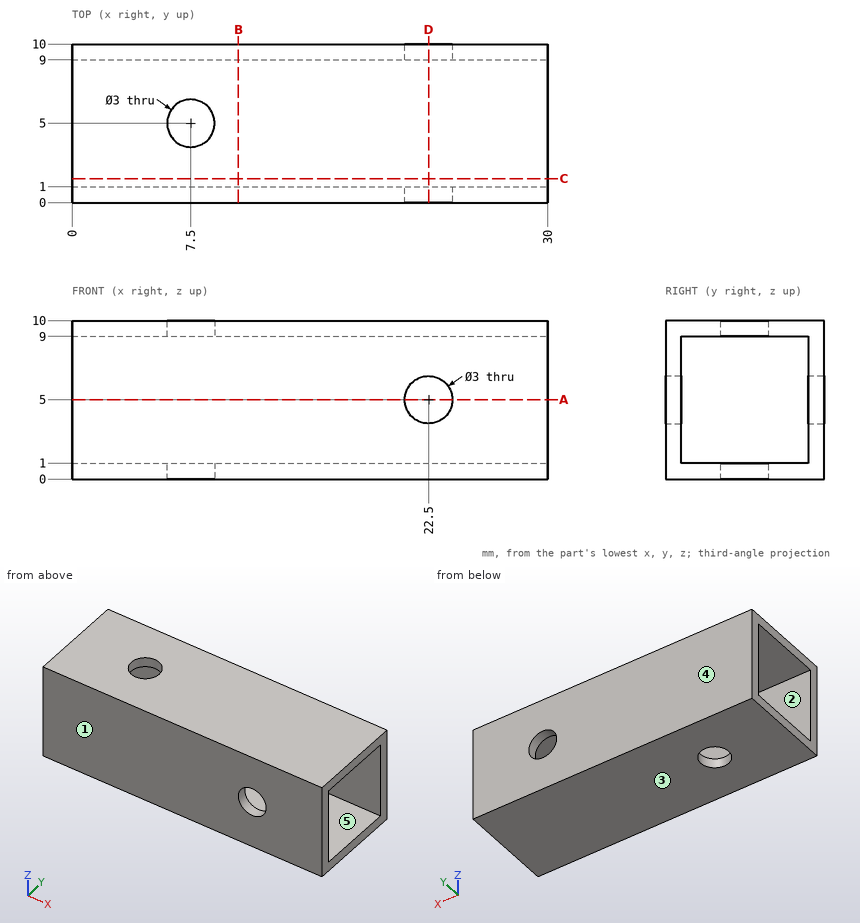
Input: dimensioned drawing with shaded views. Units: mm. Origin: part minimum x, y, z. A direction names the side the tool comes from. Round coordinates to 2 decimals unless told otherwise and drop trailing zeros. Loops run counter-clockwise (first coordinate to the right, second up) from the corner with the lowest first, then second, coordinate; pieces in that order, holes last. Notation, with made-up numbers: (49.25, 21.25) -> (98.25, 21.25) arc R31 ccw to (98.25, 53.25) -> close; hole circle Ø3 at (8.25, -26). An arc over 180 degrees is marked (long way). Use one line per item in the form item = value. Start each with the question number.
1) Section A-A on z = 5. Output: boundary loops of the cut face in (x, y).
2) Section B-B on x = 10.5. Output: boundary loops of the cut face in (y, z).
3) Section C-C on y = 1.5. Output: boundary loops of the cut face in (x, z).
4) Access query for the marked faces 4 and 5. Directions: +Z, -Z, +X, -X, +Y, -Y. A direction counts if a zero-diameter tool reaches every point of the face in a straight line with its end or side. Return the directions, or none.
5) First-contact query: P1, Ø2.5, axis at x = 22.5, z = 5, coming from the -Y side. Flat tip, straight axial feed; report the tip coordinate or a pass-through.
6) Draft query along Y for the marked faces 1, 2 and 3. Return one class per face: released by +Y, released by -Y, zero draft, split by the parting line, or undercut.
7) Line query: L1, parallel to Y at x = 7.5, z = 0.4; L2, parallel to Y at x = 17.5, z = 1.5. Output: solid intervals per line, ascending.
8) Section D-D on x = 22.5. Output: boundary loops of the cut face in (y, z).
Response:
q1.outline = (0, 0) -> (21, 0) -> (21, 1) -> (0, 1) -> close; (0, 9) -> (21, 9) -> (21, 10) -> (0, 10) -> close; (24, 0) -> (30, 0) -> (30, 1) -> (24, 1) -> close; (24, 9) -> (30, 9) -> (30, 10) -> (24, 10) -> close
q2.outline = (0, 0) -> (10, 0) -> (10, 10) -> (0, 10) -> close; hole (1, 1) -> (9, 1) -> (9, 9) -> (1, 9) -> close
q3.outline = (0, 0) -> (30, 0) -> (30, 1) -> (0, 1) -> close; (0, 9) -> (30, 9) -> (30, 10) -> (0, 10) -> close
q4.face_4 = +Z, -Z, +X, -X, +Y
q4.face_5 = +X, -X
q5.P1 = through
q6.face_1 = released by -Y
q6.face_2 = undercut
q6.face_3 = zero draft
q7.L1 = 0 to 3.5, 6.5 to 10
q7.L2 = 0 to 1, 9 to 10
q8.outline = (0, 0) -> (10, 0) -> (10, 3.5) -> (9, 3.5) -> (9, 1) -> (1, 1) -> (1, 3.5) -> (0, 3.5) -> close; (0, 6.5) -> (1, 6.5) -> (1, 9) -> (9, 9) -> (9, 6.5) -> (10, 6.5) -> (10, 10) -> (0, 10) -> close
